Design review of the part built by this model. Coordinates are the model's own, in mm. A direction names the side the tool comes from. Give positions to 0.01 mm unless a question says otherwise; leave off trailing zeros. Loops run counter-clockwise (first coordinate to the right, second up) from the corner with the lowest first, then second, coordinate; pieces in that order, holes last. Notation, with made-up numbers: (33, -27) -> (38, -27) arc R31 cw to (38, 8) -> close; hole circle Ø11 at (66, 24). An arc over 180 degrees is marked (long way). Use a Markdown table: item, result. Add a question column.
1. To check wall thickness, follow line 1 (X direction, y = -20.5, z = -2.5); line 2 (Z direction, x = -1, y = -1.5); line 3 (Z direction, x = -12, y = -12.5). State the ranges of each line that lie inside material, in increasing order.
2. Add section B-B (x = 14). State the section outline as (y, z) points, and give its area (3 significant figures).
3. Draft analysis for pull direction X (two halves, no side actions). For faces 1 (the flat face through (-5.4, 0, -11.4)), 2 (the flat face through (-22.312, -12, -4)), 3 (the flat face through (-18, -23, -4)), state which applies: pulls with the +X half, pulls with the -X half, needs draft (parallel to the pull), parting line crosses it, or undercut.
4. Add section C-C (z = -6). State the section outline as (x, y) points, and give its area (3 significant figures).
5. Add section D-D (x = 1). State the section outline as (y, z) points, and give its area (3 significant figures).
6. For faces 4 (the flat face through (13, -12, -8.127)), 5 (the flat face through (-18, -12, -8.127)), 6 (the flat face through (12, -11, -7.327)), list the 3-axis set-ups (+Z, -Z, +X, -X, +Y, -Y) from which the entire face can be reached by the end or side of a thin tool; tool diameter is ignored.
7. For pin 1 Ø3.5 at (x, y) = (-16.5, -14.5) entering from -Z; pin 2 Ø1.5 at (x, z) = (10.5, -9) entering from +Y; pin 3 Ø2 at (x, z) = (-17.5, -4.5) entering from +Y, all flat-tipped, find the tip position at first contact; note any pin that passes through.
8. Add section A-A (y = -7). State the section outline as (x, z) points, and give its area (3 significant figures).
```python
from build123d import *

# Parameters (mm, degrees)
F1_DEPTH = 25
F2_W     = 7.4
F2_H     = 7.4
F3_DEPTH = 23


with BuildPart() as f1:
    # F0 (on Front) → F1 (new body)
    with BuildSketch(Plane.XZ):
        Polygon((10.088344, -11.686348), (10.088344, -11.186348), (8.413416, -8.127029), (17.688344, -8.127029), (17.688344, 0.872971), (-22.311656, 0.872971), (-22.311656, -8.127029), (-13.036728, -8.127029), (-14.711656, -11.186348), (-14.711656, -11.686348), align=None)
    extrude(amount=F1_DEPTH)

    # F2 (on face) → F3 (cut)
    with BuildSketch(Plane(origin=(0, 0, 0), x_dir=(-1, 0, 0), z_dir=(0, 1, 0))):
        Polygon((-7.263654, -7.327029), (-7.263654, -10.886348), (10.157422, -10.886348), (10.157422, -7.327029), (13.311656, -7.327029), (13.311656, 0.072971), (-16.888344, 0.072971), (-16.888344, -7.327029), align=None)
        with Locations((17.811656, -3.627029)):
            Rectangle(F2_W, F2_H)
    extrude(amount=-F3_DEPTH, mode=Mode.SUBTRACT)


solid = f1.part
```
Taken from the geometry:
| question | item | result |
|---|---|---|
| 1 | line 1 | x = -22.31 to -21.51, -14.11 to -13.31, 16.89 to 17.69 |
| 1 | line 2 | z = -11.69 to -10.89, 0.07 to 0.87 |
| 1 | line 3 | z = -11.69 to -7.33, 0.07 to 0.87 |
| 2 | outline | (-25, -8.13) -> (0, -8.13) -> (0, -7.33) -> (-23, -7.33) -> (-23, 0.07) -> (0, 0.07) -> (0, 0.87) -> (-25, 0.87) -> close |
| 2 | area | 54.8 mm^2 |
| 3 | face 1 | needs draft |
| 3 | face 2 | pulls with the -X half |
| 3 | face 3 | undercut |
| 4 | outline | (-22.31, -25) -> (17.69, -25) -> (17.69, 0) -> (16.89, 0) -> (16.89, -23) -> (-13.31, -23) -> (-13.31, 0) -> (-14.11, 0) -> (-14.11, -23) -> (-21.51, -23) -> (-21.51, 0) -> (-22.31, 0) -> close |
| 4 | area | 135 mm^2 |
| 5 | outline | (-25, -11.69) -> (0, -11.69) -> (0, -10.89) -> (-23, -10.89) -> (-23, 0.07) -> (0, 0.07) -> (0, 0.87) -> (-25, 0.87) -> close |
| 5 | area | 61.9 mm^2 |
| 6 | face 4 | +X, +Y, -Y |
| 6 | face 5 | -X, +Y, -Y |
| 6 | face 6 | +Y |
| 7 | pin 1 | stops at z = -8.13 |
| 7 | pin 2 | passes through |
| 7 | pin 3 | stops at y = -23 |
| 8 | outline | (-22.31, -8.13) -> (-13.04, -8.13) -> (-14.71, -11.19) -> (-14.71, -11.69) -> (10.09, -11.69) -> (10.09, -11.19) -> (8.41, -8.13) -> (17.69, -8.13) -> (17.69, 0.87) -> (-22.31, 0.87) -> close; hole (-21.51, -7.33) -> (-14.11, -7.33) -> (-14.11, 0.07) -> (-21.51, 0.07) -> close; hole (-13.31, -7.33) -> (-10.16, -7.33) -> (-10.16, -10.89) -> (7.26, -10.89) -> (7.26, -7.33) -> (16.89, -7.33) -> (16.89, 0.07) -> (-13.31, 0.07) -> close |
| 8 | area | 103 mm^2 |
